Design review of the part built by this model. Coordinates are the model's own, in mm. A direction names the side the tool comes from. Round coordinates to 2 decimals unless told otherwise and drop trailing zeros. Loops run counter-clockwise (first coordinate to the right, second up) from the corner with the lowest first, then second, coordinate; pieces in that order, holes last. Notation, with made-up numbers: M 29,65 L 82,65 A13 ccw 82,80 Z; hole C 84.5,78 d9. An arc over 180 degrees is marked long. Use a Markdown table: item, result.
from build123d import *

# Parameters (mm, degrees)
F1_DEPTH = 1.5
F2_R     = 1.1
F3_DEPTH = 1.501
F4_W     = 7
F4_H     = 3
F4_R     = 3
F5_DEPTH = 1.501


with BuildPart() as f1:
    # F0 (on Top) → F1 (new body)
    with BuildSketch(Plane.XY):
        with BuildLine():
            Line((42, 3.6), (-42, 3.6))
            ThreePointArc((-42, 3.6), (-45.6, 0), (-42, -3.6))
            Line((-42, -3.6), (42, -3.6))
            ThreePointArc((42, -3.6), (45.6, 0), (42, 3.6))
        make_face()
    extrude(amount=F1_DEPTH)

    # F2 (on face) → F3 (cut, through all)
    with BuildSketch(Plane.XY.offset(1.5)):
        with Locations((-42, 0)):
            Circle(F2_R)
        with Locations((42, 0)):
            Circle(F2_R)
        Circle(F2_R)
        with Locations((-36, 0)):
            Circle(F2_R)
        with Locations((36, 0)):
            Circle(F2_R)
        with Locations((-23, 0)):
            Circle(F2_R)
        with Locations((23, 0)):
            Circle(F2_R)
        with Locations((-6, 0)):
            Circle(F2_R)
        with Locations((6, 0)):
            Circle(F2_R)
    extrude(amount=-F3_DEPTH, mode=Mode.SUBTRACT)

    # F4 (on face) → F5 (cut, through all)
    with BuildSketch(Plane.XY.offset(1.5)):
        with Locations((-33.6, 0)):
            Rectangle(F4_W, F4_H)
        with Locations((-12.1, 3.6)):
            Circle(F4_R)
        with Locations((33.6, 0)):
            Rectangle(F4_W, F4_H)
        with Locations((12.1, 3.6)):
            Circle(F4_R)
    extrude(amount=-F5_DEPTH, mode=Mode.SUBTRACT)


solid = f1.part
1. Wall thickness on line 1 along Y through (x, z) = (-6, 0.9); line 2 along X through (y, z) = (1.25, 0.3); line 3 along Y through (x, z) = (32, 1.1): over which ranges is each line inside the solid? List them lowest first. Write a range as from..to.
Check values:
| item | result |
|---|---|
| line 1 | y = -3.6..-1.1, 1.1..3.6 |
| line 2 | x = -45.38..-37.1, -30.1..-13.96, -10.24..10.24, 13.96..30.1, 37.1..45.38 |
| line 3 | y = -3.6..-1.5, 1.5..3.6 |
2. Take a section at B-B on z = 0.85. Count the separate pieces of the cut face and the enclosed holes in it, and give its area (3 significant figures).
Check values:
| item | result |
|---|---|
| separate pieces | 1 |
| enclosed holes | 9 |
| area | 549 mm² |
3. Machinability: for faces 5 (the face through (-28, 3.6, 1)), 6 (the face through (34, 1.5, 1)), which of the approach directions +Z, -Z, +X, -X, +Y, -Y give a long, thin tool a straight path to every point of the face, cutting with its end or side? Answer none if there is none.
Check values:
| item | result |
|---|---|
| face 5 | +Z, -Z, +X, -X, +Y |
| face 6 | +Z, -Z |
4. Take a section at D-D on x = 12.1. Give the boundary of the cut face in (y, z).
Check values:
| item | result |
|---|---|
| outline | M -3.6,0 L 0.6,0 L 0.6,1.5 L -3.6,1.5 Z |
5. Take a section at A-A on x = -23. Give the boundary of the cut face in (y, z), and give its area (3 significant figures).
Check values:
| item | result |
|---|---|
| outline | M -3.6,0 L -1.1,0 L -1.1,1.5 L -3.6,1.5 Z; M 1.1,0 L 3.6,0 L 3.6,1.5 L 1.1,1.5 Z |
| area | 7.50 mm² |
6. Take a section at C-C on y = 2.5. Give the boundary of the cut face in (x, z), and give its area (3 significant figures).
Check values:
| item | result |
|---|---|
| outline | M -44.59,0 L -14.89,0 L -14.89,1.5 L -44.59,1.5 Z; M -9.31,0 L 9.31,0 L 9.31,1.5 L -9.31,1.5 Z; M 14.89,0 L 44.59,0 L 44.59,1.5 L 14.89,1.5 Z |
| area | 117 mm² |
7. The part is to be moulded in two halves that separate along Y. For faces 1 (the face through (-1, -3.6, 1)), 2 (the face through (-34, -1.5, 1)), 3 (the face through (12, 0.6, 0.8)), 4 (the face through (21.9, 0, 0.8)), say which applies: pulls with the +Y half, pulls with the -Y half, needs draft (parallel to the pull), parting line crosses it, or undercut.
Check values:
| item | result |
|---|---|
| face 1 | pulls with the -Y half |
| face 2 | undercut |
| face 3 | pulls with the +Y half |
| face 4 | undercut |
8. Insertion check: pin 1 (3.5 mm diameter, centred on x = -42, y = 0, fed in from +Z). The pin has a flat end and moves straight along its axis. Give the tip position at first contact, or say it passes through.
Check values:
| item | result |
|---|---|
| pin 1 | stops at z = 1.5 |
